```python
from build123d import *

# Parameters (mm, degrees)
F0_W      = 113
F0_H      = 20
F1_DEPTH  = 3
F2_W      = 2.5
F2_H      = 20
F2_W_2    = 3
F3_DEPTH  = 12
F4_R      = 1.5
F5_DEPTH  = 3
F6_R      = 3.05
F6_R_2    = 1.5
F7_DEPTH  = 1
F8_W      = 32.75
F8_H      = 16.8
F8_W_2    = 43.6
F8_W_3    = 7.15
F9_DEPTH  = 3
F10_SIZE  = 5
F11_ANGLE = 180


# Not quite as in the source:
# - a feature of the source that left no trace in its solid (it failed there, or was rolled back) is left out


with BuildPart() as f1:
    # F0 (on Top) → F1 (new body)
    with BuildSketch(Plane.XY):
        Rectangle(F0_W, F0_H)
    extrude(amount=F1_DEPTH)

    # F2 (on face) → F3 (join)
    with BuildSketch(Plane.XY.offset(3)):
        with Locations((-10.25, 0)):
            Rectangle(F2_W, F2_H)
        with Locations((37, 0)):
            Rectangle(F2_W_2, F2_H)
    extrude(amount=-F3_DEPTH)

    # F4 (on face) → F5 (cut, through all)
    with BuildSketch(Plane.XY.offset(3)):
        with Locations((-51.1, 0)):
            Circle(F4_R)
        with Locations((43.1, 0)):
            Circle(F4_R)
    extrude(amount=-F5_DEPTH, mode=Mode.SUBTRACT)

    # F6 (on face) → F7 (cut)
    with BuildSketch(Plane.XY.offset(3)):
        with Locations((-51.1, 0)):
            Circle(F6_R)
        with Locations((-51.1, 0)):
            Circle(F6_R_2, mode=Mode.SUBTRACT)
        with Locations((43.1, 0)):
            Circle(F6_R)
        with Locations((43.1, 0)):
            Circle(F6_R_2, mode=Mode.SUBTRACT)
    extrude(amount=-F7_DEPTH, mode=Mode.SUBTRACT)

    # F8 (on face) → F9 (cut, through all)
    with BuildSketch(Plane.XY.offset(3)):
        with Locations((-30.075, 0)):
            Rectangle(F8_W, F8_H)
        with Locations((13.5, 0)):
            Rectangle(F8_W_2, F8_H)
        with Locations((51.325, 0)):
            Rectangle(F8_W_3, F8_H)
    extrude(amount=-F9_DEPTH, mode=Mode.SUBTRACT)

    # F10
    f10_edges = [f1.edges().sort_by_distance(p)[0] for p in [
        (-56.5, 10, 1.5),
        (-56.5, -10, 1.5),
    ]]
    chamfer(f10_edges, length=F10_SIZE)


with BuildPart() as f1_1:
    # F11: moved
    add(f1.part.rotate(Axis((2.5, -10, 3), (-1, 0, 0)), F11_ANGLE))


solid = f1_1.part
```
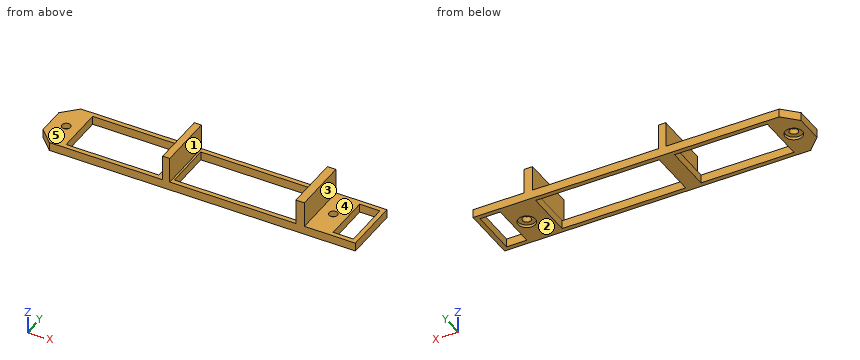
The listing builds one solid part. Answer for the finished solid, in the listing's coordinates (mm). Face numbers are marked on the shaded views. A direction names the side the tool comes from. Give positions to 0.01 mm unless a question says otherwise; leave off trailing zeros. Order: outer loops, then holes, each group sorted by start corner. A loop starts at its lowest first (then second) coordinate and runs counter-clockwise, first axis right, second up. Notation, with made-up numbers: M -34,87.5 L -30,87.5 A27 cw -30,109.5 Z; hole C 22,38.25 d6. An arc over 180 degrees is marked long. Put each result on its own line as item: value. Start each with the question number.
Item 1: The part is cut by section B-B, the plane x = 26. Determine the outline of the cut face in (y, z), and give its area (3 significant figures).
Item 2: Which of the six approach directions +Z, -Z, +X, -X, +Y, -Y give full straight-line access (tool end or side, diameter ignored) to the marked faces 4 and 5?
Item 3: The part is cut by section C-C, the plane y = -16. Determine the outline of the cut face in (x, z), and give its area (3 significant figures).
Item 4: For a pull along X with two mould halves and no side action, classify the marked faces 1, 2 and 3 as +X half, -X half, draft (parallel to the pull), parting line (faces both ways), or undercut.
Item 5: The part is cut by section A-A, the plane z = 10.25. Determine the outline of the cut face in (x, y), and give its area (3 significant figures).
Item 6: Find the intervals of material crossed by line 1 along X through (y, z) = (-20, 3.5); line 2 along X through (y, z) = (-20, 5.45); line 3 along Y through (x, z) = (43.1, 3.5), in increasing order.
Item 7: The part is cut by section D-D, the plane x = 43.1. Determine the outline of the cut face in (y, z), and give its area (3 significant figures).
Item 8: Flat-ended cylindrical pins translate along their axes: P1, Ø4.5, axis at y = -24, z = 11.5, coming from the +X side; P2, Ø1, axis at y = -20.5, z = 7, coming from the -X side; P3, Ø5, axis at x = 43.1, y = -20, coming from the +Z side. Find the tip coordinate at first contact, or state that the pin passes through.
Answer key:
1. outline: M -30,3 L -28.4,3 L -28.4,6 L -30,6 Z; M -11.6,3 L -10,3 L -10,6 L -11.6,6 Z
1. area: 9.60 mm²
2. face 4: +Z, +X, +Y, -Y
2. face 5: +Z, -X, +Y, -Y
3. outline: M -56.5,3 L -46.45,3 L -46.45,6 L -56.5,6 Z; M -13.7,3 L -8.3,3 L -8.3,6 L -9,6 L -9,15 L -11.5,15 L -11.5,6 L -13.7,6 Z; M 35.3,3 L 47.75,3 L 47.75,6 L 38.5,6 L 38.5,15 L 35.5,15 L 35.5,6 L 35.3,6 Z; M 54.9,3 L 56.5,3 L 56.5,6 L 54.9,6 Z
3. area: 138 mm²
4. face 1: undercut
4. face 2: draft
4. face 3: +X half
5. outline: M -11.5,-30 L -9,-30 L -9,-10 L -11.5,-10 Z; M 35.5,-30 L 38.5,-30 L 38.5,-10 L 35.5,-10 Z
5. area: 110 mm²
6. line 1: x = -56.5 to -54.15, -48.05 to -46.45, -13.7 to -8.3, 35.3 to 40.05, 46.15 to 47.75, 54.9 to 56.5
6. line 2: x = -56.5 to -52.6, -49.6 to -46.45, -13.7 to -8.3, 35.3 to 41.6, 44.6 to 47.75, 54.9 to 56.5
6. line 3: y = -30 to -23.05, -16.95 to -10
7. outline: M -30,3 L -23.05,3 L -23.05,4 L -21.5,4 L -21.5,6 L -30,6 Z; M -18.5,4 L -16.95,4 L -16.95,3 L -10,3 L -10,6 L -18.5,6 Z
7. area: 47.9 mm²
8. P1: stops at x = 38.5
8. P2: stops at x = -11.5
8. P3: stops at z = 6
